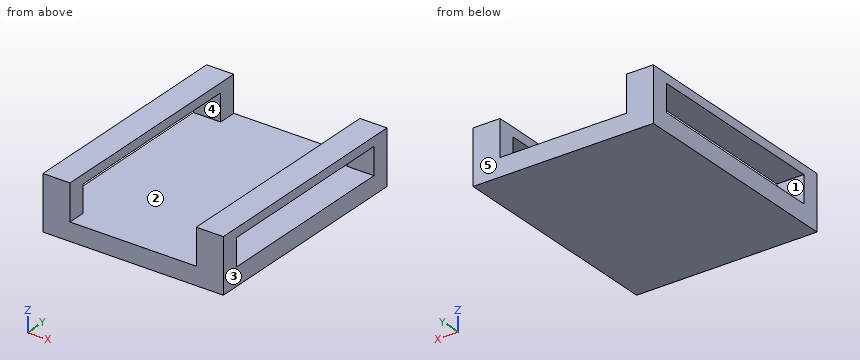
from build123d import *

# Parameters (mm, degrees)
F0_W     = 20
F0_H     = 25
F1_DEPTH = 2
F2_W     = 3
F2_H     = 25
F3_DEPTH = 4
F4_W     = 21
F4_H     = 3
F5_DEPTH = 25


with BuildPart() as f1:
    # F0 (on Top) → F1 (new body)
    with BuildSketch(Plane.XY):
        Rectangle(F0_W, F0_H)
    extrude(amount=F1_DEPTH)

    # F2 (on face) → F3 (join)
    with BuildSketch(Plane.XY.offset(2)):
        with Locations((-8.5, 0)):
            Rectangle(F2_W, F2_H)
        with Locations((8.5, 0)):
            Rectangle(F2_W, F2_H)
    extrude(amount=F3_DEPTH)

    # F4 (on face) → F5 (cut)
    with BuildSketch(Plane.YZ.offset(10)):
        with Locations((0, 3.5)):
            Rectangle(F4_W, F4_H)
    extrude(amount=-F5_DEPTH, mode=Mode.SUBTRACT)


solid = f1.part
Model file for the job. Use its own axes, mm. Face numbers are marked on the shaded views. A direction names the side the tool comes from. Give positions to 0.01 mm unless a question says otherwise; leave off trailing zeros. Order: outer loops, then holes, each group sorted by start corner. A loop starts at its lowest first (then second) coordinate and runs counter-clockwise, first axis right, second up. Notation, with made-up numbers: (69, -8) - (96, -8) arc R14 ccw to (96, 9) - close; hole circle Ø1 at (5, 71). An arc over 180 degrees is marked (long way). Write item = value, one per line. Start each with the question number.
1. Drop a flat-ended pin along its axis: P1, Ø10, axis at x = 0.5, y = -4, coming from the +Z side. Give the stop position or say it passes through.
2. Cut at B-B, the plane y = -0.25. List the corners of the cut face in (x, z), and give its area (3 significant figures).
3. Cut at D-D, the plane z = 5.3. List the corners of the cut face in (x, y).
4. Cut at A-A, the plane z = 4. List the corners of the cut face in (x, y).
5. Which spindle directions (+Z, -Z, +X, -X, +Y, -Y) get a long thin tool onto all of the face, cutting with end or side? Do the marked faces 4 and 5. Say none if no direction does.
6. Cut at C-C, the plane x = -8.5. List the corners of the cut face in (y, z), and give its area (3 significant figures).
7. Probe line 1 along X through (y, z) = (-11.5, 3.75); line 2 along Y through (x, z) = (-8, 3.85); line 3 along Z through (x, y) = (-7.5, -7.5). List the from-to ranges inside material, lowest first.
8. Two-plate mould, pull along X, no slides. Class the marked faces 1, 2 and 3: pulls with the +X half, pulls with the -X half, needs draft (parallel to the pull), parting line crosses it, or undercut.
Taken from the geometry:
q1.P1 = 2
q2.outline = (-10, 0) - (10, 0) - (10, 2) - (-10, 2) - close; (-10, 5) - (-7, 5) - (-7, 6) - (-10, 6) - close; (7, 5) - (10, 5) - (10, 6) - (7, 6) - close
q2.area = 46.0 mm²
q3.outline = (-10, -12.5) - (-7, -12.5) - (-7, 12.5) - (-10, 12.5) - close; (7, -12.5) - (10, -12.5) - (10, 12.5) - (7, 12.5) - close
q4.outline = (-10, -12.5) - (-7, -12.5) - (-7, -10.5) - (-10, -10.5) - close; (-10, 10.5) - (-7, 10.5) - (-7, 12.5) - (-10, 12.5) - close; (7, -12.5) - (10, -12.5) - (10, -10.5) - (7, -10.5) - close; (7, 10.5) - (10, 10.5) - (10, 12.5) - (7, 12.5) - close
q5.face_4 = +X, -X
q5.face_5 = +Z, -Z, +X, -X, +Y
q6.outline = (-12.5, 0) - (12.5, 0) - (12.5, 6) - (-12.5, 6) - close; hole (-10.5, 2) - (10.5, 2) - (10.5, 5) - (-10.5, 5) - close
q6.area = 87.0 mm²
q7.line_1 = -10 to -7, 7 to 10
q7.line_2 = -12.5 to -10.5, 10.5 to 12.5
q7.line_3 = 0 to 2, 5 to 6
q8.face_1 = needs draft
q8.face_2 = undercut
q8.face_3 = pulls with the +X half
